from build123d import *

# Parameters (mm, degrees)
SKETCH1_W               = 254
SKETCH1_H               = 203.2
BOSS_EXTRUDE1_DEPTH     = 5.588
F_1_4_CLEARANCE_HOLE1_D = 7.14248
FILLET1_R               = 2.54


with BuildPart() as part:
    # Sketch1 → Boss-Extrude1 (new body)
    with BuildSketch(Plane.XY):
        Rectangle(SKETCH1_W, SKETCH1_H)
        with BuildLine():
            Line((-102.092252, 88.9), (-102.092252, -88.9))
            ThreePointArc((-102.092252, -88.9), (-104.619552, -91.4273), (-107.146852, -88.9))
            Line((-107.146852, -88.9), (-107.146852, 88.9))
            ThreePointArc((-107.146852, 88.9), (-104.619552, 91.4273), (-102.092252, 88.9))
        make_face(mode=Mode.SUBTRACT)
        with BuildLine():
            Line((107.146852, 88.9), (107.146852, -88.9))
            ThreePointArc((107.146852, -88.9), (104.619552, -91.4273), (102.092252, -88.9))
            Line((102.092252, -88.9), (102.092252, 88.9))
            ThreePointArc((102.092252, 88.9), (104.619552, 91.4273), (107.146852, 88.9))
        make_face(mode=Mode.SUBTRACT)
    extrude(amount=BOSS_EXTRUDE1_DEPTH)

    # 1/4 Clearance Hole1 (through all)
    with Locations(Plane.XY.offset(5.588)):
        with Locations((0, 0)):
            Hole(F_1_4_CLEARANCE_HOLE1_D / 2)

    # Fillet1
    fillet1_edges = [part.edges().sort_by_distance(p)[0] for p in [
        (127, -101.6, 2.794),
        (-127, -101.6, 2.794),
        (-127, 101.6, 2.794),
        (127, 101.6, 2.794),
    ]]
    fillet(fillet1_edges, radius=FILLET1_R)


solid = part.part
Can you work these out from the model? Positions are in its coordinate system, mm. A direction names the side the tool comes from. Round coordinates to 2 decimals unless told otherwise and drop trailing zeros. Order: outer loops, then holes, each group sorted by start corner. A loop starts at its lowest first (then second) coordinate and runs counter-clockwise, first axis right, second up. Notation, with made-up numbers: (16, -36.75) - (66, -36.75) arc R32 ccw to (66, -3.75) - close; hole circle Ø11 at (89.25, -10.75). An arc over 180 degrees is marked (long way). Answer in a Markdown table with one row per item.
(1) If we mould it in two halves opening along X, with no side actions, what happens to faces 3 (the face through (102.092, -1, 3)), 4 (the face through (-127, -1, 3)), 5 (the face through (-102.092, 1, 3)), 6 (the face through (-2, 24, 5.588))? For each: released by +X, released by -X, zero draft, split by the parting line, or undercut.
From the geometry:
| item | result |
|---|---|
| face 3 | undercut |
| face 4 | released by -X |
| face 5 | undercut |
| face 6 | zero draft |
(2) Suppose I cut it at A-A, the plane y = 50. Please give me the cut outline in (x, z).
From the geometry:
| item | result |
|---|---|
| outline | (-127, 0) - (-107.15, 0) - (-107.15, 5.59) - (-127, 5.59) - close; (-102.09, 0) - (102.09, 0) - (102.09, 5.59) - (-102.09, 5.59) - close; (107.15, 0) - (127, 0) - (127, 5.59) - (107.15, 5.59) - close |
(3) For P1, Ø6.5, axis at x = 0, y = 0, coming from the -Z side, with a flat end and sliding along its axis, tell me the tip position at first contact or that it passes through.
From the geometry:
| item | result |
|---|---|
| P1 | passes through |
(4) Suppose I cut it at D-D, the plane x = 0. Please give me the cut outline in (y, z).
From the geometry:
| item | result |
|---|---|
| outline | (-101.6, 0) - (-3.57, 0) - (-3.57, 5.59) - (-101.6, 5.59) - close; (3.57, 0) - (101.6, 0) - (101.6, 5.59) - (3.57, 5.59) - close |
(5) Suppose I cut it at C-C, the plane y = 0. Please give me the cut outline in (x, z), plus the area to 3 significant figures.
From the geometry:
| item | result |
|---|---|
| outline | (-127, 0) - (-107.15, 0) - (-107.15, 5.59) - (-127, 5.59) - close; (-102.09, 0) - (-3.57, 0) - (-3.57, 5.59) - (-102.09, 5.59) - close; (3.57, 0) - (102.09, 0) - (102.09, 5.59) - (3.57, 5.59) - close; (107.15, 0) - (127, 0) - (127, 5.59) - (107.15, 5.59) - close |
| area | 1,320 mm2 |
(6) Please list where these lines run through material, in increasing order: L1, parallel to X at y = -80.5, z = 3.85; L2, parallel to Y at x = 0, z = 2.4; L3, parallel to X at y = -90, z = 4.85. Write a range as from..to.
From the geometry:
| item | result |
|---|---|
| L1 | x = -127..-107.15, -102.09..102.09, 107.15..127 |
| L2 | y = -101.6..-3.57, 3.57..101.6 |
| L3 | x = -127..-106.89, -102.34..102.34, 106.89..127 |
(7) Suppose I cut it at B-B, the plane z = 1.35. Please give me the cut outline in (x, y), plus the area to 3 significant figures.
From the geometry:
| item | result |
|---|---|
| outline | (-127, -99.06) arc R2.54 ccw to (-124.46, -101.6) - (124.46, -101.6) arc R2.54 ccw to (127, -99.06) - (127, 99.06) arc R2.54 ccw to (124.46, 101.6) - (-124.46, 101.6) arc R2.54 ccw to (-127, 99.06) - close; hole (-107.15, -88.9) arc R2.53 ccw to (-102.09, -88.9) - (-102.09, 88.9) arc R2.53 ccw to (-107.15, 88.9) - close; hole circle Ø7.14 at (0, 0); hole (102.09, -88.9) arc R2.53 ccw to (107.15, -88.9) - (107.15, 88.9) arc R2.53 ccw to (102.09, 88.9) - close |
| area | 49,700 mm2 |
(8) Which directions (+Z, -Z, +X, -X, +Y, -Y) give clear straight access to the entire face, cutting with the end or side of a thin tool? Please do faces 1 (the face through (-104.564, -91.427, 2.755)), 2 (the face through (127, -1, 3)).
From the geometry:
| item | result |
|---|---|
| face 1 | +Z, -Z |
| face 2 | +Z, -Z, +X, +Y, -Y |
